Geometry: final body of the model. Coordinates: model frame, mm. Face numbers are marked on the shaded views. Give positions to 0.01 mm unless a question says otherwise; leave off trailing zeros. Write each loop counter-clockwise with the first axis right and the second up, starting at its lowest first coordinate (ties: lowest second). Pieces come first, ordered by that corner, then holes. Notation, with made-up numbers: (7.25, 43.25) -> (23.25, 43.25) arc R6 cw to (23.25, 49.25) -> close; hole circle Ø3 at (55.5, 89.5). An arc over 180 degrees is marked (long way). Answer in a Markdown table with one row per item. Add a question column.
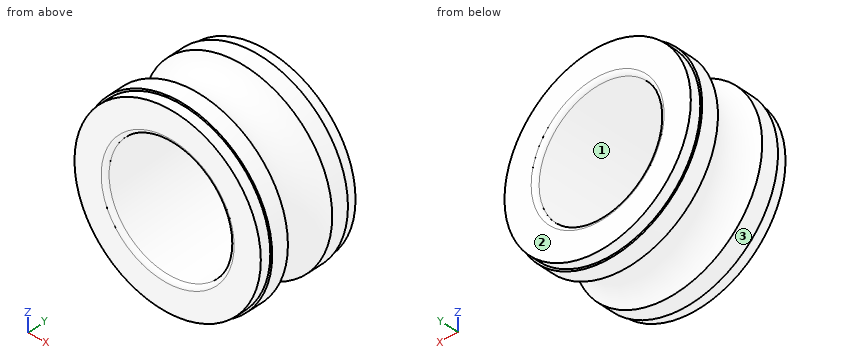
from build123d import *


with BuildPart() as part:
    # Sketch1 → Revolve1 (revolve)
    with BuildSketch(Plane(origin=(0, 0, 0), x_dir=(-1, 0, 0), z_dir=(0, 0, -1))):
        with BuildLine():
            Line((-4.575, -0.5), (-4.575, -1.330865705))
            ThreePointArc((-4.575, -1.330865705), (-3.9, -2.5), (-4.575, -3.669134295))
            Line((-4.575, -3.669134295), (-4.575, -4.5))
            Line((-4.575, -4.5), (-4.4835, -4.5))
            Line((-4.4835, -4.5), (-4.4835, -5))
            Line((-4.4835, -5), (-3.2, -5))
            ThreePointArc((-3.2, -5), (-3.058578644, -4.941421356), (-3, -4.8))
            Line((-3, -4.8), (-3, -0.2))
            ThreePointArc((-3, -0.2), (-3.058578644, -0.058578644), (-3.2, 0))
            Line((-3.2, 0), (-4.4835, 0))
            Line((-4.4835, 0), (-4.4835, -0.5))
            Line((-4.4835, -0.5), (-4.575, -0.5))
        make_face()
    revolve(axis=Axis((0, -5.003495744, 0), (0, 1, 0)))


solid = part.part
Q1. Section D-D on y = -2.15. Return loops of the section in (x, z), and give its area (3 significant figures).
Q2. Section C-C on y = -3.8. Return loops of the section in (x, z) (3 decimals).
Q3. Contact query for a flat-ended pin moving along its axis: pin 1 Ø3 at (x, y) = (-1.5, -3) entering from -Z. Output: stop coordinate, or through.
Q4. Pull-direction query (X, two-part tool) for the marked faces 1, 2 and 3; classes: +X half, -X half, draft (parallel to the pull), parting line (faces both ways), or undercut.
Q5. Line query: probe 1 along Z at (x, y) = (0, -4.4) (3 decimals); probe 2 along Y at (x, z) = (-3.5, 2); probe 3 along Y at (x, z) = (0.25, 4.25). Output: solid intervals per line, ascending. Write a range as from..to.
Checks:
| question | item | result |
|---|---|---|
| 1 | outline | circle Ø7.89 at (0, 0); hole circle Ø6 at (0, 0) |
| 1 | area | 20.6 mm^2 |
| 2 | outline | circle Ø9.15 at (0, 0); hole circle Ø6 at (0, 0) |
| 3 | pin 1 | z = -4.57 |
| 4 | face 1 | undercut |
| 4 | face 2 | draft |
| 4 | face 3 | parting line |
| 5 | probe 1 | -4.575..-3, 3..4.575 |
| 5 | probe 2 | -5..-3.08, -1.92..0 |
| 5 | probe 3 | -5..-3.41, -1.59..0 |
